```python
from build123d import *

# Parameters (mm, degrees)
SKETCH1_W           = 42.3
SKETCH1_H           = 42.3
BOSS_EXTRUDE1_DEPTH = 37.4396
CHAMFER1_SIZE       = 5.08
SKETCH2_R           = 11.43
SKETCH2_R_2         = 11
CUT_EXTRUDE1_DEPTH  = 1.27
BOSS_EXTRUDE2_START = 2.54
SKETCH3_R           = 11
SKETCH3_R_2         = 3.81
BOSS_EXTRUDE2_DEPTH = 2.54
SKETCH4_R           = 2.5
BOSS_EXTRUDE3_DEPTH = 21.9202
CUT_EXTRUDE2_REACH  = 49.92
SKETCH5_R           = 1.5


with BuildPart() as part:
    # Sketch1 → Boss-Extrude1 (new body)
    with BuildSketch(Plane(origin=(0, 0, 0), x_dir=(1, 0, 0), z_dir=(0, 1, 0))):
        Rectangle(SKETCH1_W, SKETCH1_H)
    extrude(amount=BOSS_EXTRUDE1_DEPTH)

    # Chamfer1
    chamfer1_edges = [part.edges().sort_by_distance(p)[0] for p in [
        (21.15, 18.7198, 21.15),
        (-21.15, 18.7198, 21.15),
        (-21.15, 18.7198, -21.15),
        (21.15, 18.7198, -21.15),
    ]]
    chamfer(chamfer1_edges, length=CHAMFER1_SIZE)

    # Sketch2 → Cut-Extrude1 (cut)
    with BuildSketch(Plane(origin=(0, 37.4396, 0), x_dir=(1, 0, 0), z_dir=(0, 1, 0))):
        with Locations(Location((0, 0, 0), (0, 0, 270))):
            Circle(SKETCH2_R)
        with Locations(Location((0, 0, 0), (0, 0, 270))):
            Circle(SKETCH2_R_2, mode=Mode.SUBTRACT)
    extrude(amount=-CUT_EXTRUDE1_DEPTH, mode=Mode.SUBTRACT)

    # Sketch3 → Boss-Extrude2 (add)
    with BuildSketch(Plane(origin=(0, 37.4396, 0), x_dir=(1, 0, 0), z_dir=(0, 1, 0)).offset(BOSS_EXTRUDE2_START)):
        with Locations(Location((0, 0, 0), (0, 0, 270))):
            Circle(SKETCH3_R)
        with Locations(Location((0, 0, 0), (0, 0, 270))):
            Circle(SKETCH3_R_2, mode=Mode.SUBTRACT)
    extrude(amount=-BOSS_EXTRUDE2_DEPTH)

    # Sketch4 → Boss-Extrude3 (add)
    with BuildSketch(Plane(origin=(0, 37.4396, 0), x_dir=(1, 0, 0), z_dir=(0, 1, 0))):
        with Locations(Location((0, 0, 0), (0, 0, 90))):
            Circle(SKETCH4_R)
    extrude(amount=BOSS_EXTRUDE3_DEPTH)

    # Sketch5 → Cut-Extrude2 (cut, up to next)
    with BuildSketch(Plane(origin=(0, 37.4396, 0), x_dir=(1, 0, 0), z_dir=(0, 1, 0)), mode=Mode.PRIVATE) as cut_extrude2_sk1:
        with Locations(Location((15.5, 15.5, 0), (0, 0, 270))):
            Circle(SKETCH5_R)
    cut_extrude2_tool1 = extrude(cut_extrude2_sk1.sketch, amount=-CUT_EXTRUDE2_REACH, mode=Mode.PRIVATE) & part.part
    # Sketch5 → Cut-Extrude2 (cut, up to next)
    with BuildSketch(Plane(origin=(0, 37.4396, 0), x_dir=(1, 0, 0), z_dir=(0, 1, 0)), mode=Mode.PRIVATE) as cut_extrude2_sk2:
        with Locations(Location((15.5, -15.5, 0), (0, 0, 270))):
            Circle(SKETCH5_R)
    cut_extrude2_tool2 = extrude(cut_extrude2_sk2.sketch, amount=-CUT_EXTRUDE2_REACH, mode=Mode.PRIVATE) & part.part
    # Sketch5 → Cut-Extrude2 (cut, up to next)
    with BuildSketch(Plane(origin=(0, 37.4396, 0), x_dir=(1, 0, 0), z_dir=(0, 1, 0)), mode=Mode.PRIVATE) as cut_extrude2_sk3:
        with Locations(Location((-15.5, -15.5, 0), (0, 0, 270))):
            Circle(SKETCH5_R)
    cut_extrude2_tool3 = extrude(cut_extrude2_sk3.sketch, amount=-CUT_EXTRUDE2_REACH, mode=Mode.PRIVATE) & part.part
    # Sketch5 → Cut-Extrude2 (cut, up to next)
    with BuildSketch(Plane(origin=(0, 37.4396, 0), x_dir=(1, 0, 0), z_dir=(0, 1, 0)), mode=Mode.PRIVATE) as cut_extrude2_sk4:
        with Locations(Location((-15.5, 15.5, 0), (0, 0, 270))):
            Circle(SKETCH5_R)
    cut_extrude2_tool4 = extrude(cut_extrude2_sk4.sketch, amount=-CUT_EXTRUDE2_REACH, mode=Mode.PRIVATE) & part.part
    add(cut_extrude2_tool1.solids().sort_by_distance((15.5, 37.4396, -15.5))[0], mode=Mode.SUBTRACT)
    add(cut_extrude2_tool2.solids().sort_by_distance((15.5, 37.4396, 15.5))[0], mode=Mode.SUBTRACT)
    add(cut_extrude2_tool3.solids().sort_by_distance((-15.5, 37.4396, 15.5))[0], mode=Mode.SUBTRACT)
    add(cut_extrude2_tool4.solids().sort_by_distance((-15.5, 37.4396, -15.5))[0], mode=Mode.SUBTRACT)


solid = part.part
```
The model under review builds one solid part; all positions refer to its coordinate system, in mm. A direction names the side the tool comes from. Round coordinates to 2 decimals unless told otherwise and drop trailing zeros. Write each loop counter-clockwise with the first axis right and the second up, starting at its lowest first coordinate (ties: lowest second). Pieces come first, ordered by that corner, then holes. Notation, with made-up numbers: (60, -14.5) - (64, -14.5) arc R17 cw to (64, 0.5) - close; hole circle Ø5 at (11.25, 44.5). An arc over 180 degrees is marked (long way). Answer as CSV lines item,"result". Start each with the question number.
(1) We need section A-A on y = 16.5. State the section outline as (x, z) points, plus the area to 3 significant figures.
(2) For faces 4 (the flat face through (0, 59.36, 0)), 5 (the flat face through (6, 36.17, -9.4)), list the 3-axis set-ups (+Z, -Z, +X, -X, +Y, -Y) from which the entire face can be reached by the end or side of a thin tool; tool diameter is ignored.
(3) We need section B-B on z = 10. State the section outline as (x, y) points.
(4) For pin 1 Ø10 at (x, z) = (15.5, -13) entering from -Y; pin 2 Ø4 at (x, z) = (15.5, 15.5) entering from +Y; pin 3 Ø7 at (x, z) = (3.5, -5) entering from +Y, all flat-tipped, find the tip position at first contact; note any pin that passes through.
(5) We need section D-D on z = 0. State the section outline as (x, y) points.
(6) To check wall thickness, follow line 1 (X direction, y = 26, z = 15.5); line 2 (X direction, y = 38, z = 0); line 3 (Z direction, x = 6, y = 37). State the ranges of each line that lie inside material, in increasing order.
(7) We need section C-C on x = -6. State the section outline as (y, z) points, plus the area to 3 significant figures.
(8) Draft analysis for pull direction Z (two halves, no side actions). For faces 1 (the flat face through (0, 18, -21.15)), 2 (the flat face through (21.15, 18, 0)), 3 (the cylindrical face through (-10.74, 38.1, -2.38)), state which applies: pulls with the +Z half, pulls with the -Z half, needs draft (parallel to the pull), parting line crosses it, or undercut.
Worked answers:
1,outline,"(-21.15, -16.07) - (-16.07, -21.15) - (16.07, -21.15) - (21.15, -16.07) - (21.15, 16.07) - (16.07, 21.15) - (-16.07, 21.15) - (-21.15, 16.07) - close; hole circle Ø3 at (-15.5, -15.5); hole circle Ø3 at (-15.5, 15.5); hole circle Ø3 at (15.5, -15.5); hole circle Ø3 at (15.5, 15.5)"
1,area,"1,710 mm²"
2,face 4,"+Z, -Z, +X, -X, +Y"
2,face 5,"+Y"
3,outline,"(-21.15, 0) - (21.15, 0) - (21.15, 37.44) - (5.54, 37.44) - (5.54, 36.17) - (4.58, 36.17) - (4.58, 39.98) - (-4.58, 39.98) - (-4.58, 36.17) - (-5.54, 36.17) - (-5.54, 37.44) - (-21.15, 37.44) - close"
4,pin 1,"y = 0"
4,pin 2,"y = 37.44"
4,pin 3,"y = 39.98"
5,outline,"(-21.15, 0) - (21.15, 0) - (21.15, 37.44) - (11.43, 37.44) - (11.43, 36.17) - (11, 36.17) - (11, 39.98) - (3.81, 39.98) - (3.81, 37.44) - (2.5, 37.44) - (2.5, 59.36) - (-2.5, 59.36) - (-2.5, 37.44) - (-3.81, 37.44) - (-3.81, 39.98) - (-11, 39.98) - (-11, 36.17) - (-11.43, 36.17) - (-11.43, 37.44) - (-21.15, 37.44) - close"
6,line 1,"-21.15 to -17, -14 to 14, 17 to 21.15"
6,line 2,"-11 to -3.81, -2.5 to 2.5, 3.81 to 11"
6,line 3,"-21.15 to -9.73, -9.22 to 9.22, 9.73 to 21.15"
7,outline,"(0, -21.15) - (37.44, -21.15) - (37.44, -9.73) - (36.17, -9.73) - (36.17, -9.22) - (39.98, -9.22) - (39.98, 9.22) - (36.17, 9.22) - (36.17, 9.73) - (37.44, 9.73) - (37.44, 21.15) - (0, 21.15) - close"
7,area,"1,630 mm²"
8,face 1,"pulls with the -Z half"
8,face 2,"needs draft"
8,face 3,"undercut"
